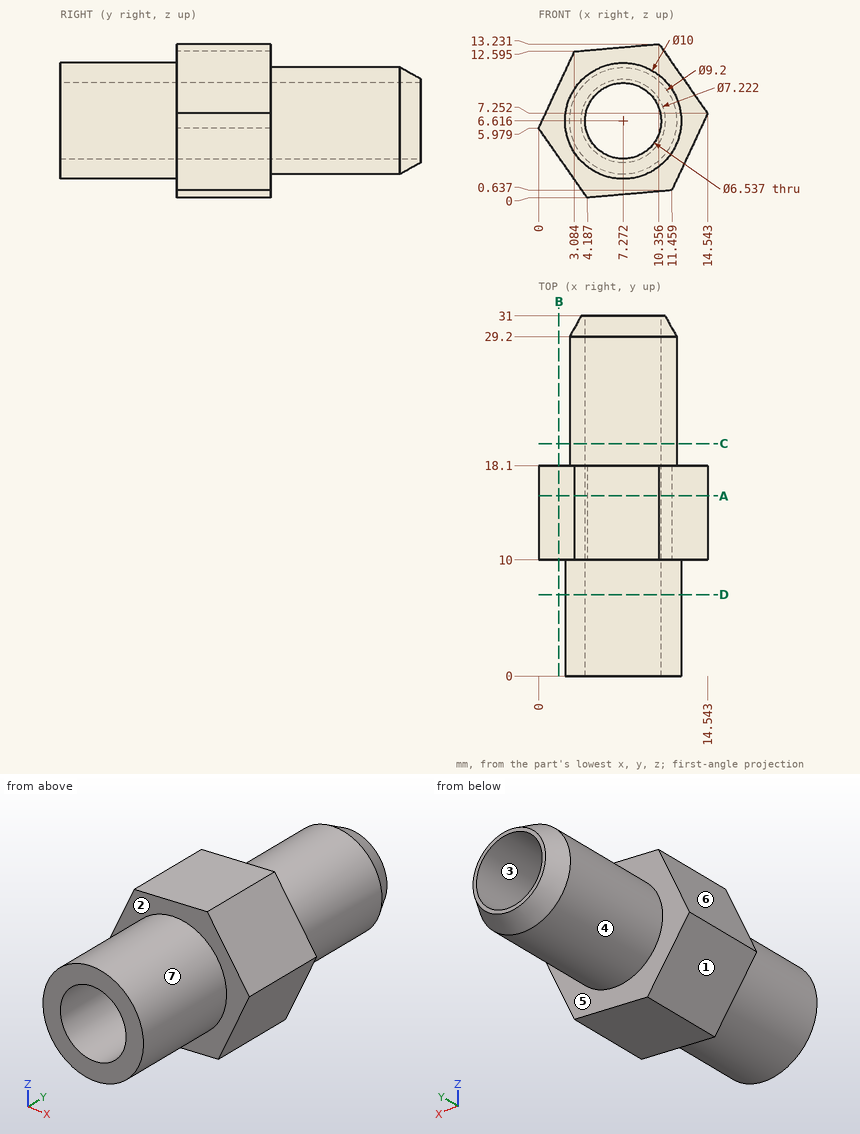
Drawing for the job (mm, zero at the part's lowest x, y, z). A direction names the side the tool comes from. Round coordinates to 2 decimals unless told otherwise and drop trailing zeros. Write each loop counter-clockwise with the first axis right and the second up, starting at its lowest first coordinate (ties: lowest second). Pieces come first, ordered by that corner, then holes. Notation, with made-up numbers: M -1.75,-4 L 12.25,-4 A12 ccw 12.25,1 Z; hole C 65,-16.5 d3. An arc over 180 degrees is marked long. Answer as a JSON object with one key per item and string values. Group by question number.
(1) Cut at D-D (y = 7). Give the cut face in (x, z) (1 decimal).
(2) Cut at A-A (y = 15.5). Give the cut face in (x, z) (1 decimal), and give its area (3 significant figures).
(3) Cut at B-B (x = 1.75). Give the cut face in (y, z).
(4) Cut at C-C (y = 20). Give the cut face in (x, z) (1 decimal).
(5) Which spindle directions (+Z, -Z, +X, -X, +Y, -Y) get a long thin tool onto all of the face, cutting with end or side? Do the marked faces 5, 6 and 7. Say none if no direction does.
(6) Drill centre lines: L1, parallel to Z at x = 7.25, y = 18.5 (1 decimal); L2, parallel to Z at x = 5.25, y = 16 (1 decimal); L3, parallel to X at y = 28.5, z = 9.25 (1 decimal). Where is each one in solid material? Low to high.
(7) Flat gauge pins, fed straight in: pin 1 (3 mm diameter, centred on x = 5.5, z = 4.5, fed in from +Y); pin 2 (2 mm diameter, centred on x = 11.5, y = 4, fed in from +Z) (1 decimal); pin 3 (3 mm diameter, centred on y = 13, z = 5.5, fed in from +X) (1 decimal); pin 4 (1 mm diameter, centred on x = 3.5, z = 9.5, fed in from +Y). Where does each tip first touch, or does it go through?
(8) Mould opens along Z. For the marked faces 1, 2, 3 and 4 say: pulls with the +Z half, pulls with the -Z half, needs draft (parallel to the pull), parting line crosses it, or undercut.
Responses:
{
 "1": {"outline": "C 7.3,6.6 d10; hole C 7.3,6.6 d6.5"},
 "2": {"outline": "M 0,6 L 4.2,0 L 11.5,0.6 L 14.5,7.3 L 10.4,13.2 L 3.1,12.6 Z; hole C 7.3,6.6 d6.5", "area": "105 mm2"},
 "3": {"outline": "M 10,3.48 L 18.1,3.48 L 18.1,9.73 L 10,9.73 Z"},
 "4": {"outline": "C 7.3,6.6 d9.2; hole C 7.3,6.6 d6.5"},
 "5": {"face 5": "+Y", "face 6": "+Z, -X, +Y, -Y", "face 7": "-Y"},
 "6": {"L1": "z = 2 to 3.3, 9.9 to 11.2", "L2": "z = 0.1 to 4, 9.2 to 12.8", "L3": "x = 3.5 to 5.3, 9.2 to 11"},
 "7": {"pin 1": "stops at y = 31", "pin 2": "stops at z = 10.4", "pin 3": "stops at x = 14.4", "pin 4": "stops at y = 29.84"},
 "8": {"face 1": "pulls with the -Z half", "face 2": "needs draft", "face 3": "undercut", "face 4": "parting line crosses it"}
}
